from build123d import *

# Parameters (mm, degrees)
RESSALTO_EXTRUS_O1_DEPTH = 2


with BuildPart() as part:
    # Esboço1 → Ressalto-extrusão1 (new body)
    with BuildSketch(Plane(origin=(0, 0, 0), x_dir=(0, 0, -1), z_dir=(1, 0, 0))):
        with BuildLine():
            Line((0, 0), (0, 25))
            ThreePointArc((0, 25), (-0.292893219, 25.707106781), (-1, 26))
            Line((-1, 26), (-2, 26))
            Line((-2, 26), (-2, 15.5))
            ThreePointArc((-2, 15.5), (-3.5, 14), (-5, 15.5))
            Line((-5, 15.5), (-5, 25))
            ThreePointArc((-5, 25), (-5.292893219, 25.707106781), (-6, 26))
            Line((-6, 26), (-70, 26))
            ThreePointArc((-70, 26), (-71.248507537, 26.141106905), (-72.434027777, 26.557308768))
            ThreePointArc((-72.434027777, 26.557308768), (-72.519947834, 26.593984538), (-72.608915487, 26.622482343))
            ThreePointArc((-72.608915487, 26.622482343), (-93.139545948, 26.696407833), (-111, 16.571367926))
            Line((-111, 16.571367926), (-109, 16.571367926))
            ThreePointArc((-109, 16.571367926), (-107, 14.571367926), (-109, 12.571367926))
            Line((-109, 12.571367926), (-113.466213279, 12.571367926))
            ThreePointArc((-113.466213279, 12.571367926), (-113.800393506, 12.443286702), (-113.963364883, 12.124662231))
            ThreePointArc((-113.963364883, 12.124662231), (-113.460397939, 8.860641338), (-111.403723296, 6.276671998))
            ThreePointArc((-111.403723296, 6.276671998), (-111.106614108, 5.923183177), (-111, 5.473893017))
            Line((-111, 5.473893017), (-111, -1))
            ThreePointArc((-111, -1), (-110.707106781, -1.707106781), (-110, -2))
            Line((-110, -2), (-102.358378421, -2))
            ThreePointArc((-102.358378421, -2), (-101.544115198, -1.580495826), (-101.413025617, -0.673950808))
            ThreePointArc((-101.413025617, -0.673950808), (-86.793753315, 21.176788674), (-69.688908754, 1.211763478))
            ThreePointArc((-69.688908754, 1.211763478), (-69.489971865, 0.372211611), (-68.711587809, 0))
            Line((-68.711587809, 0), (0, 0))
        make_face()
        with BuildLine():
            Line((-105, 8), (-105, 2))
            ThreePointArc((-105, 2), (-107, 0), (-109, 2))
            Line((-109, 2), (-109, 8))
            ThreePointArc((-109, 8), (-107, 10), (-105, 8))
        make_face(mode=Mode.SUBTRACT)
        with BuildLine():
            Line((-58.816829377, 22.236628683), (-56, 16.938943126))
            ThreePointArc((-56, 16.938943126), (-56.82695206, 14.234104814), (-59.531790371, 15.061056874))
            Line((-59.531790371, 15.061056874), (-62.348619748, 20.358742432))
            ThreePointArc((-62.348619748, 20.358742432), (-61.521667688, 23.063580743), (-58.816829377, 22.236628683))
        make_face(mode=Mode.SUBTRACT)
    extrude(amount=RESSALTO_EXTRUS_O1_DEPTH)


solid = part.part
Geometry: final body of the model. Coordinates: model frame, mm. A direction names the side the tool comes from. Round coordinates to 2 decimals unless told otherwise and drop trailing zeros. Write each loop counter-clockwise with the first axis right and the second up, starting at its lowest first coordinate (ties: lowest second). Pieces come first, ordered by that corner, then holes. Notation, with made-up numbers: M 24.5,25 L 62.5,25 A15 cw 62.5,35 Z; hole C 15,11.25 d11. An arc over 180 degrees is marked long. Write item = value, one per line.
Item 1: Material intervals for line 1 along Y through (x, z) = (0.5, 108.5); line 2 along Z through (x, y) = (0.3, 15); line 3 along Z through (x, y) = (1.65, 3), sorted ascending. Write a range as [from, to].
Findings:
line_1 = [-2, 0.68], [9.32, 12.63], [16.51, 18.82]
line_2 = [0, 2.09], [4.91, 56.03], [59.5, 72.92], [98.71, 107.05]
line_3 = [0, 69.4], [102.23, 105], [109, 111]
Item 2: Pin query (flat end, axial travel): P1, Ø0.6, axis at x = 1.5, z = 51.5, coming from the -Y side; P2, Ø0.5, axis at x = 1, z = 1.5, coming from the +Y side. Return the tip coordinate at first contact, or that it passes through.
Findings:
P1 = 0
P2 = 26
Item 3: Section query A-A on x = 0.65. State how many separate pieces and enclosed holes the cut face has, then the cut area to 3 significant figures.
Findings:
separate_pieces = 1
enclosed_holes = 2
area = 2,190 mm^2
Item 4: Section query C-C on z = 3.5. Return loops of the section in (x, y), then the cut area to 3 significant figures.
Findings:
outline = M 0,0 L 2,0 L 2,14 L 0,14 Z
area = 28.0 mm^2
Item 5: Pull-direction query (Y, two-part tool) for faces 5 (the face through (1, 21, 2)), 6 (the face through (0.986, 19.625, 57.428)), 7 (the face through (1, 14, 3.5)); classes: pulls with the +Y half, pulls with the -Y half, needs draft (parallel to the pull), parting line crosses it, or undercut.
Findings:
face_5 = needs draft
face_6 = undercut
face_7 = pulls with the +Y half
Item 6: Section query B-B on z = 15. Return loops of the section in (x, y).
Findings:
outline = M 0,0 L 2,0 L 2,26 L 0,26 Z
Item 7: Access query for faces 1 (the face through (1, 0, 35)), 2 (the face through (1, 12.571, 111)), 3 (the face through (1, 0, 107)), 4 (the face through (1, 26, 38)). Directions: +Z, -Z, +X, -X, +Y, -Y. A direction counts if a zero-diameter tool reaches every point of the face in a straight line with its end or side. Return the directions, or none.
Findings:
face_1 = -Z, +X, -X, -Y
face_2 = +Z, +X, -X
face_3 = +X, -X
face_4 = -Z, +X, -X, +Y
